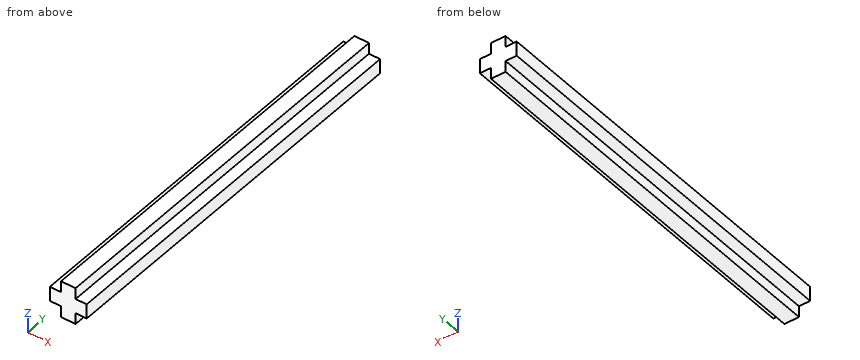
from build123d import *

# Parameters (mm, degrees)
F0_W     = 0.89
F0_H     = 0.89
F1_DEPTH = 23.72


with BuildPart() as f1:
    # F0 (on Front) → F1 (new body, symmetric)
    with BuildSketch(Plane.XZ):
        Polygon((-0.89, 0.89), (-2.25, 0.89), (-2.25, -0.89), (-0.89, -0.89), (-0.89, 0), align=None)
        Polygon((-0.89, 2.25), (-0.89, 0.89), (0, 0.89), (0.89, 0.89), (0.89, 2.25), align=None)
        with Locations((-0.445, 0.445)):
            Rectangle(F0_W, F0_H)
        with Locations((0.445, 0.445)):
            Rectangle(F0_W, F0_H)
        with Locations((-0.445, -0.445)):
            Rectangle(F0_W, F0_H)
        Polygon((0, -0.89), (-0.89, -0.89), (-0.89, -2.25), (0.89, -2.25), (0.89, -0.89), align=None)
        Polygon((2.25, 0.89), (0.89, 0.89), (0.89, 0), (0.89, -0.89), (2.25, -0.89), align=None)
        with Locations((0.445, -0.445)):
            Rectangle(F0_W, F0_H)
    extrude(amount=F1_DEPTH, both=True)


solid = f1.part
Geometry: final body of the model. Coordinates: model frame, mm. Give positions to 0.01 mm unless a question says otherwise; leave off trailing zeros. Loops run counter-clockwise (first coordinate to the right, second up) from the corner with the lowest first, then second, coordinate; pieces in that order, holes last. Notation, with made-up numbers: M -1.75,-2 L 31.25,-2 A10 cw 31.25,8 Z; hole C 89,78 d7. An arc over 180 degrees is marked long. Put each result on its own line as item: value. Start each with the question number.
1) Ray query, line 1 along X through (y, z) = (-13, 1.4). Return the intervals inside material, ascending.
2) Cut plane B-B (x = 1.4). Output: boundary loops of the cut face in (y, z).
3) Cut plane C-C (z = 1.7). Output: boundary loops of the cut face in (x, y), then the cut area to 3 significant figures.
4) Cut plane A-A (y = 17.5). Output: boundary loops of the cut face in (x, z), then the cut area to 3 significant figures.
5) Contact query for flat-ended pins moving along their axis: pin 1 (0.7 mm diameter, centred on x = -2, y = 11, fed in from +Z); pin 2 (0.7 mm diameter, centred on y = 6.5, z = -1.5, fed in from -X); pin 3 (0.7 mm diameter, centred on x = -1.5, y = 10.5, fed in from -Z). Output: stop coordinate, or through.
Verdict:
1. line 1: -0.89 to 0.89
2. outline: M -23.72,-0.89 L 23.72,-0.89 L 23.72,0.89 L -23.72,0.89 Z
3. outline: M -0.89,-23.72 L 0.89,-23.72 L 0.89,23.72 L -0.89,23.72 Z
3. area: 84.4 mm2
4. outline: M -2.25,-0.89 L -0.89,-0.89 L -0.89,-2.25 L 0.89,-2.25 L 0.89,-0.89 L 2.25,-0.89 L 2.25,0.89 L 0.89,0.89 L 0.89,2.25 L -0.89,2.25 L -0.89,0.89 L -2.25,0.89 Z
4. area: 12.9 mm2
5. pin 1: z = 0.89
5. pin 2: x = -0.89
5. pin 3: z = -0.89
